Part print with two shaded views. Sizes in mm from the minimum x, y, z corner. Give positions to 0.01 mm unless a question says otherwise; leave off trailing zeros. Loops run counter-clockwise (first coordinate to the right, second up) from the corner with the lowest first, then second, coordinate; pieces in that order, holes last. Notation, with made-up numbers: M -6.5,73 L 10.5,73 A19 cw 10.5,81 Z; hole C 33.5,-35 d7. An arc over 180 degrees is marked long. Answer as a JSON object with one key per item and string values. Group by question number.
1. Slice it at C-C (y = 3.35). Give the number of separate pieces and of enclosed holes in the cut face, then the cut area to 3 significant figures.
2. Slice it at A-A (z = 51.5). List the corners of the cut face in (x, y).
3. Slice it at D-D (x = 199). List the corners of the cut face in (y, z).
4. Drop flat-ended pins along their axis: pin 1 Ø5 at (x, z) = (150, 158) entering from -Y; pin 2 Ø2.5 at (x, z) = (158, 150) entering from -Y; pin 3 Ø2 at (x, y) = (99.5, 4.5) entering from +Z. Give the stop position or say it passes through.
5. Slice it at B-B (z = 200). List the corners of the cut face in (x, y), then the cut area to 3 significant figures.
6. Drill centre lines: line 1 along X through (y, z) = (3.9, 150); line 2 along X through (y, z) = (4.4, 203) (1 decimal); line 3 along Z through (x, y) = (142, 1.35). Where is each one in solid material? Low to high. Write a range as [from, to].
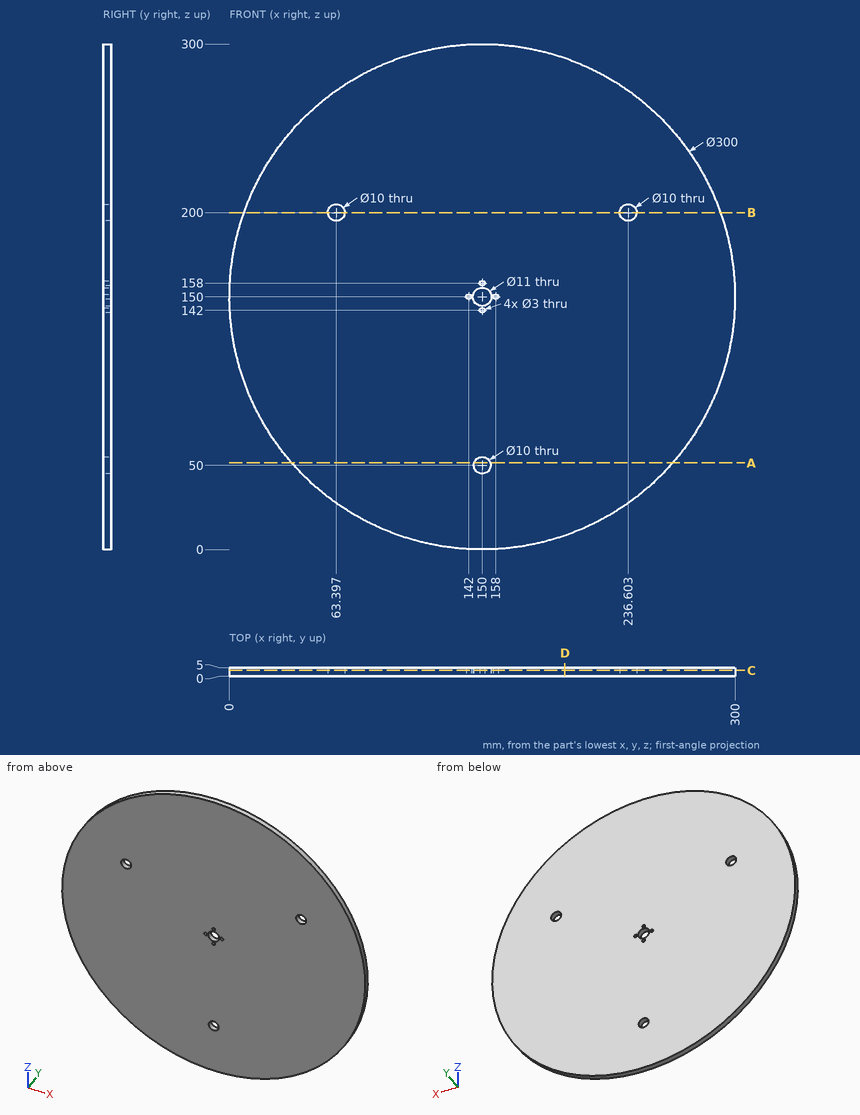
Established:
{
 "1": {"separate pieces": "1", "enclosed holes": "8", "area": "70,300 mm^2"},
 "2": {"outline": "M 36.87,0 L 145.23,0 L 145.23,5 L 36.87,5 Z; M 154.77,0 L 263.13,0 L 263.13,5 L 154.77,5 Z"},
 "3": {"outline": "M 0,8.23 L 5,8.23 L 5,291.77 L 0,291.77 Z"},
 "4": {"pin 1": "stops at y = 0", "pin 2": "passes through", "pin 3": "stops at z = 291.6"},
 "5": {"outline": "M 8.58,0 L 58.4,0 L 58.4,5 L 8.58,5 Z; M 68.4,0 L 231.6,0 L 231.6,5 L 68.4,5 Z; M 241.6,0 L 291.42,0 L 291.42,5 L 241.6,5 Z", "area": "1,310 mm^2"},
 "6": {"line 1": "x = [0, 140.5], [143.5, 144.5], [155.5, 156.5], [159.5, 300]", "line 2": "x = [9.7, 59.4], [67.4, 232.6], [240.6, 290.3]", "line 3": "z = [0.21, 148.5], [151.5, 299.79]"}
}
